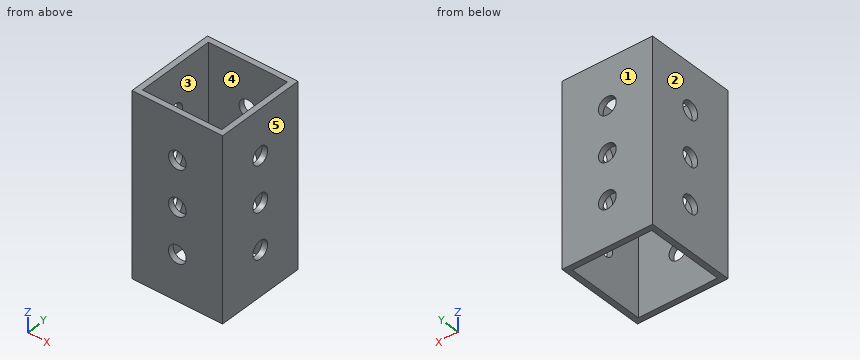
```python
from build123d import *

# Parameters (mm, degrees)
SKETCH1_W           = 25.4
SKETCH1_H           = 25.4
SKETCH1_W_2         = 22.225
SKETCH1_H_2         = 22.225
BOSS_EXTRUDE1_DEPTH = 50.8
SKETCH2_R           = 2.4892
CUT_EXTRUDE1_DEPTH  = 26.4
SKETCH3_R           = 2.4892
CUT_EXTRUDE2_DEPTH  = 26.4


with BuildPart() as part:
    # Sketch1 → Boss-Extrude1 (new body)
    with BuildSketch(Plane.XY):
        with Locations((12.7, 12.7)):
            Rectangle(SKETCH1_W, SKETCH1_H)
        with Locations((12.7, 12.7)):
            Rectangle(SKETCH1_W_2, SKETCH1_H_2, mode=Mode.SUBTRACT)
    extrude(amount=BOSS_EXTRUDE1_DEPTH)

    # Sketch2 → Cut-Extrude1 (cut, through all)
    with BuildSketch(Plane(origin=(0, 25.4, 0), x_dir=(1, 0, 0), z_dir=(0, 1, 0))):
        with Locations((12.7, -12.7)):
            Circle(SKETCH2_R)
        with Locations((12.7, -25.4)):
            Circle(SKETCH2_R)
        with Locations((12.7, -38.1)):
            Circle(SKETCH2_R)
    extrude(amount=-CUT_EXTRUDE1_DEPTH, mode=Mode.SUBTRACT)

    # Sketch3 → Cut-Extrude2 (cut, through all)
    with BuildSketch(Plane.ZY):
        with Locations((12.7, 12.7)):
            Circle(SKETCH3_R)
        with Locations((25.4, 12.7)):
            Circle(SKETCH3_R)
        with Locations((38.1, 12.7)):
            Circle(SKETCH3_R)
    extrude(amount=-CUT_EXTRUDE2_DEPTH, mode=Mode.SUBTRACT)


solid = part.part
```
Design review of the part built by this model. Coordinates are the model's own, in mm. Face numbers are marked on the shaded views. A direction names the side the tool comes from. Coordinates: 2 decimals unless noted, no trailing zeros. Loops run counter-clockwise (first coordinate to the right, second up) from the corner with the lowest first, then second, coordinate; pieces in that order, holes last. Notation, with made-up numbers: (33.25, 56) - (88.25, 56) arc R16 ccw to (88.25, 73) - close; hole circle Ø1 at (73, -38.75). An arc over 180 degrees is marked (long way). Use CSV: the item, a comma, the result in double quotes. Start each with the question number.
1) Consider section A-A on z = 25.4. Write out the cut boundary in (x, y), then the cut area to 3 significant figures.
2) Consider section B-B on x = 12.7. Give the number of separate pieces and of enclosed holes in the cut face, then the cut area to 3 significant figures.
3) Tool access review of the marked faces 4 and 5: name each direction out of +Z, -Z, +X, -X, +Y, -Y from which nothing blocks a thin tool from reaching the whole face with its end or side.
4) The part is to be moulded in two halves that separate along Y. For the marked faces 1, 2 and 3, say which applies: +Y half, -Y half, draft (parallel to the pull), parting line (faces both ways), or undercut.
5) For pin 1 Ø5 at (x, z) = (10, 12.5) entering from -Y, flat-tipped, find the tip position at first contact; note if it passes through.
6) Wall thickness on L1, parallel to Z at x = 12.7, y = 24.5; L2, parallel to X at y = 23.5, z = 28: over which ranges is each line inside the solid? List them lowest first. Write a range as from..to.
7) Consider section D-D on x = 4. Write out the cut boundary in (y, z).
Geometry says:
1,outline,"(0, 0) - (10.21, 0) - (10.21, 1.59) - (1.59, 1.59) - (1.59, 10.21) - (0, 10.21) - close; (0, 15.19) - (1.59, 15.19) - (1.59, 23.81) - (10.21, 23.81) - (10.21, 25.4) - (0, 25.4) - close; (15.19, 0) - (25.4, 0) - (25.4, 10.21) - (23.81, 10.21) - (23.81, 1.59) - (15.19, 1.59) - close; (15.19, 23.81) - (23.81, 23.81) - (23.81, 15.19) - (25.4, 15.19) - (25.4, 25.4) - (15.19, 25.4) - close"
1,area,"120 mm^2"
2,separate pieces,"8"
2,enclosed holes,"0"
2,area,"114 mm^2"
3,face 4,"+Z, -Z"
3,face 5,"+Z, -Z, +X, +Y, -Y"
4,face 1,"+Y half"
4,face 2,"draft"
4,face 3,"undercut"
5,pin 1,"y = 0"
6,L1,"0..10.21, 15.19..22.91, 27.89..35.61, 40.59..50.8"
6,L2,"0..1.59, 23.81..25.4"
7,outline,"(0, 0) - (1.59, 0) - (1.59, 50.8) - (0, 50.8) - close; (23.81, 0) - (25.4, 0) - (25.4, 50.8) - (23.81, 50.8) - close"
